The listing builds one solid part. Answer for the finished solid, in the listing's coordinates (mm). Coordinates: 2 decimals unless noted, no trailing zeros. One line per item, written item: value. Start each with the question number.
Q1. Straight lines are drawn through the part: line 1 along Y through (x, z) = (11, 109); line 2 along X through (y, z) = (73, -131); line 3 along Z through (x, y) = (-29, 15). For each, find the intervals that lie inside material, in ascending order. Write a range as [from, to].
Q2. Determine the mould class of faces 1 (the flat face through (-4, 0, 0)), 2 (the flat face through (-4, 2.54, 0)) for opening direction Z: pulls with the +Z half, pulls with the -Z half, needs draft (parallel to the pull), parting line crosses it, or undercut.
Q3. Each of these flat-tipped pins is pushed along its axis until it touches: pin 1 Ø10 at (x, y) = (-113, 30.5) entering from -Z; pin 2 Ø10 at (x, z) = (37.5, 110.5) entering from +Y; pin 3 Ø1.5 at (x, y) = (-40.5, 49) entering from -Z. Where does it stop, or does it pass through?
```python
from build123d import *

# Parameters (mm, degrees)
SKETCH1_W           = 304.8
SKETCH1_H           = 304.8
BOSS_EXTRUDE1_DEPTH = 76.2
BOSS_EXTRUDE1_TAPER = -10
FILLET2_R           = 25.4
SHELL1_T            = -2.54


with BuildPart() as part:
    # Sketch1 → Boss-Extrude1 (new body)
    with BuildSketch(Plane(origin=(0, 0, 0), x_dir=(1, 0, 0), z_dir=(0, 1, 0))):
        Rectangle(SKETCH1_W, SKETCH1_H)
    extrude(amount=BOSS_EXTRUDE1_DEPTH, taper=BOSS_EXTRUDE1_TAPER)

    # Fillet2
    fillet2_edges = [part.edges().sort_by_distance(p)[0] for p in [
        (0, 0, 152.4),
        (-152.4, 0, 0),
        (0, 0, -152.4),
        (152.4, 0, 0),
        (159.118057965, 38.1, 159.118057965),
        (-159.118057965, 38.1, 159.118057965),
        (-159.118057965, 38.1, -159.118057965),
        (159.118057965, 38.1, -159.118057965),
    ]]
    fillet(fillet2_edges, radius=FILLET2_R)

    # Shell1
    shell1_openings = [part.faces().sort_by_distance(p)[0] for p in [
        (0, 76.2, 0),
    ]]
    offset(amount=SHELL1_T, openings=shell1_openings, kind=Kind.INTERSECTION)


solid = part.part
```
Output:
1. line 1: y = [0, 2.54]
1. line 2: x = [-165.27, -162.69], [162.69, 165.27]
1. line 3: z = [-154.26, -151.44], [151.44, 154.26]
2. face 1: needs draft
2. face 2: undercut
3. pin 1: stops at z = -158.66
3. pin 2: stops at y = 2.54
3. pin 3: stops at z = -161.17
